```python
from build123d import *

# Parameters (mm, degrees)
SKETCH2_R          = 1.0414
CUT_EXTRUDE1_DEPTH = 16.998643219
FILLET1_R          = 0.127


with BuildPart() as part:
    # Sketch1 → Revolve1 (revolve)
    with BuildSketch(Plane(origin=(0, 0, 0), x_dir=(0, 0, -1), z_dir=(1, 0, 0)), mode=Mode.PRIVATE) as revolve1_sk:
        Polygon((-7.1247, 0), (-7.1247, 2.2733), (-6.5532, 2.2733), (-6.5532, 4.8895), (0, 5.1435), (6.5532, 4.8895), (6.5532, 2.2733), (7.1247, 2.2733), (7.1247, 0), align=None)
    revolve(revolve1_sk.sketch.rotate(Axis((0, 0, 7.1247), (0, 0, -1)), 90), axis=Axis((0, 0, 7.1247), (0, 0, -1)))

    # Sketch2 → Cut-Extrude1 (cut, through all)
    with BuildSketch(Plane.XY.offset(7.1247)):
        Circle(SKETCH2_R)
    extrude(amount=-CUT_EXTRUDE1_DEPTH, mode=Mode.SUBTRACT)

    # Fillet1
    fillet1_edges = [part.edges().sort_by_distance(p)[0] for p in [
        (-4.8895, 0, 6.5532),
        (-4.8895, 0, -6.5532),
    ]]
    fillet(fillet1_edges, radius=FILLET1_R)


solid = part.part
```
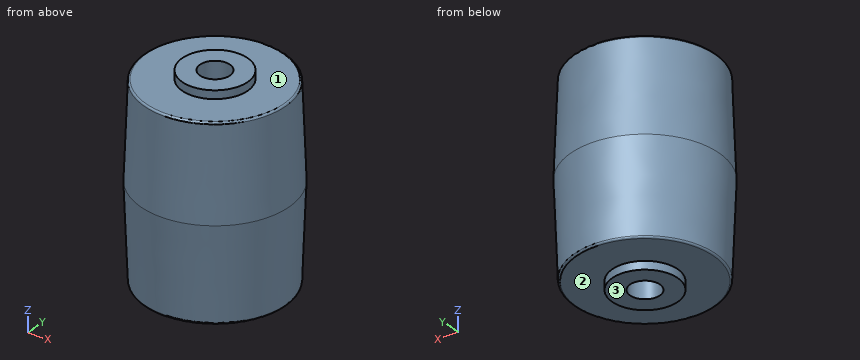
For this review, take the finished solid that the model builds, in its own axes (mm). Face numbers are marked on the shaded views. A direction names the side the tool comes from. Round coordinates to 2 decimals unless told otherwise and drop trailing zeros. Write each loop counter-clockwise with the first axis right and the second up, starting at its lowest first coordinate (ties: lowest second). Pieces come first, ordered by that corner, then holes. Notation, with made-up numbers: M -1.5,55 L 19.5,55 A20 cw 19.5,90 Z; hole C 50.5,22.5 d2. An arc over 180 degrees is marked long. One line per item, written item: value. Start each with the question number.
(1) We need section C-C (z = -2.5). Give the boundary of the cut face in (x, y).
(2) We need section A-A (y = 0). Give the boundary of the cut face in (x, z).
(3) Machinability: for the marked faces 1, 2 and 3, which of the approach directions +Z, -Z, +X, -X, +Y, -Y give a long, thin tool a straight path to every point of the face, cutting with its end or side? Answer none if there is none.
(4) Insertion check: pin 1 (1.5 mm diameter, centred on x = 3.5, y = -4, fed in from +Z); pin 2 (3 mm diameter, centred on x = -1.5, z = -4.5, fed in from +Y). Each pin has a flat end and moves straight along its axis. Give the tip position at first contact, or say it passes through.
(5) We need section D-D (z = 4.25). Give the boundary of the cut face in (x, y).
(6) Wall thickness on line 1 (Z direction, x = 3, y = -1); line 2 (Y direction, x = -0.25, z = -1.75); line 3 (Y direction, x = -0.5, z = 1.5): over which ranges is each line inside the solid? List them lowest first.
Result:
1. outline: C 0,0 d10.09; hole C 0,0 d2.08
2. outline: M -5.14,0 L -4.89,-6.43 A0.13 ccw -4.77,-6.55 L -2.27,-6.55 L -2.27,-7.12 L -1.04,-7.12 L -1.04,7.12 L -2.27,7.12 L -2.27,6.55 L -4.77,6.55 A0.13 ccw -4.89,6.43 Z; M 1.04,-7.12 L 2.27,-7.12 L 2.27,-6.55 L 4.77,-6.55 A0.13 ccw 4.89,-6.43 L 5.14,0 L 4.89,6.43 A0.13 ccw 4.77,6.55 L 2.27,6.55 L 2.27,7.12 L 1.04,7.12 Z
3. face 1: +Z
3. face 2: -Z
3. face 3: -Z, +X, -X, +Y, -Y
4. pin 1: z = 6.55
4. pin 2: y = 5
5. outline: C 0,0 d9.96; hole C 0,0 d2.08
6. line 1: -6.55 to 6.55
6. line 2: -5.07 to -1.01, 1.01 to 5.07
6. line 3: -5.06 to -0.91, 0.91 to 5.06
